```python
from build123d import *

# Parameters (mm, degrees)
PAD_DEPTH       = 10
SKETCH001_R     = 1.75
POCKET_DEPTH    = 15.001
SKETCH002_R     = 4
POCKET001_DEPTH = 5
SKETCH005_R     = 4
SKETCH005_R_2   = 2.25
POCKET002_DEPTH = 9
SKETCH006_W     = 6.5
SKETCH006_H     = 2
POCKET003_DEPTH = 9
FILLET_R        = 3
FILLET001_R     = 3


with BuildPart() as part:
    # Sketch → Pad (new body)
    with BuildSketch(Plane.XY):
        Polygon((-5, 11), (5, 11), (5, -11), (-5, -11), (-10, -2.5), (-10, 2.5), align=None)
    extrude(amount=PAD_DEPTH)

    # Sketch001 → Pocket (cut, through all)
    with BuildSketch(Plane.YZ.offset(5)):
        with Locations((-6, 5)):
            Circle(SKETCH001_R)
        with Locations((6, 5)):
            Circle(SKETCH001_R)
    extrude(amount=-POCKET_DEPTH, mode=Mode.SUBTRACT)

    # Sketch002 → Pocket001 (cut)
    with BuildSketch(Plane(origin=(-10, 0, 0), x_dir=(0, -1, 0), z_dir=(-1, 0, 0))):
        with Locations((-6, 5)):
            Circle(SKETCH002_R)
        with Locations((6, 5)):
            Circle(SKETCH002_R)
    extrude(amount=-POCKET001_DEPTH, mode=Mode.SUBTRACT)

    # Sketch005 → Pocket002 (cut)
    with BuildSketch(Plane.XY.offset(10)):
        Circle(SKETCH005_R)
        Circle(SKETCH005_R_2, mode=Mode.SUBTRACT)
    extrude(amount=-POCKET002_DEPTH, mode=Mode.SUBTRACT)

    # Sketch006 → Pocket003 (cut)
    with BuildSketch(Plane.XY.offset(10)):
        with Locations((-6.75, 0)):
            Rectangle(SKETCH006_W, SKETCH006_H)
    extrude(amount=-POCKET003_DEPTH, mode=Mode.SUBTRACT)

    # Fillet
    fillet_edges = [part.edges().sort_by_distance(p)[0] for p in [
        (-3.872983, 1, 5.5),
    ]]
    fillet(fillet_edges, radius=FILLET_R)

    # Fillet001
    fillet001_edges = [part.edges().sort_by_distance(p)[0] for p in [
        (-3.872983, -1, 5.5),
    ]]
    fillet(fillet001_edges, radius=FILLET001_R)


solid = part.part
```
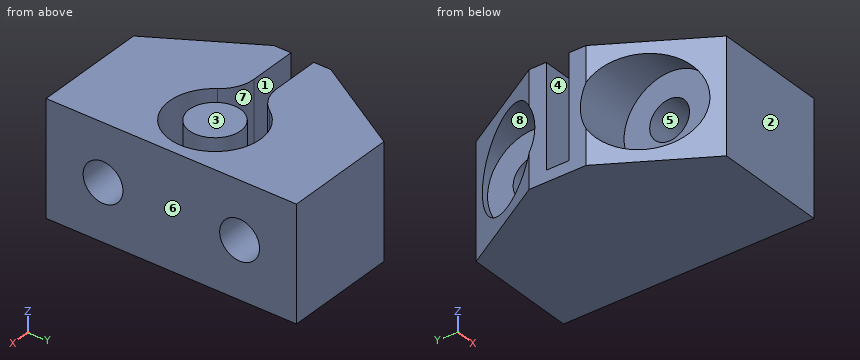
Model file for the job. Use its own axes, mm. Face numbers are marked on the shaded views. A direction names the side the tool comes from. Give positions to 0.01 mm unless a question says otherwise; leave off trailing zeros. Loops run counter-clockwise (first coordinate to the right, second up) from the corner with the lowest first, then second, coordinate; pieces in that order, holes last. Notation, with made-up numbers: (-24.75, 39) - (29.25, 39) arc R29 ccw to (29.25, 69) - close; hole circle Ø11 at (39, 67). An arc over 180 degrees is marked (long way). One line per item, written item: value. Start each with the question number.
1. Pull direction Y, two halves, no side cores. Call the marked faces 1, 2 and 3: pulls with the +Y half, pulls with the -Y half, needs draft (parallel to the pull), parting line crosses it, or undercut.
2. Slice it at C-C (x = -1). List the corners of the cut face in (y, z), plus the area to 3 significant figures.
3. Which spindle directions (+Z, -Z, +X, -X, +Y, -Y) get a long thin tool onto all of the face, cutting with end or side? Do the marked faces 4, 5, 6, 7 and 8. Say none if no direction does.
4. Slice it at D-D (z = 1.25). List the corners of the cut face in (x, y).
5. Slice it at A-A (y = 0). List the corners of the cut face in (x, z).
6. Pin check, flat tips, straight feed: pin 1 (4.5 mm diameter, centred on x = -8.5, z = 7.5, fed in from +Y); pin 2 (3 mm diameter, centred on y = 6, z = 5, fed in from +X); pin 3 (3.5 mm diameter, centred on x = -7, z = 7, fed in from -Y) (3 decimals); pin 4 (5.5 mm diameter, centred on y = -6, z = 5, fed in from -X). Stop position of each tip, or through.
7. Probe L1, parallel to Y at x = -8.2, z = 5; L2, parallel to Y at x = 0.75, z = 6.5; L3, parallel to Z at x = -2.25, y = 6. List the from-to ranges inside material, lowest first. Write a range as from..to.
8. Slice it at B-B (z = 6.5). List the corners of the cut face in (x, y), plus the area to 3 significant figures.
Solution:
1. face 1: undercut
1. face 2: pulls with the -Y half
1. face 3: needs draft
2. outline: (-11, 0) - (11, 0) - (11, 10) - (3.87, 10) - (3.87, 1) - (2.02, 1) - (2.02, 10) - (-2.02, 10) - (-2.02, 1) - (-3.87, 1) - (-3.87, 10) - (-11, 10) - close; hole circle Ø3.5 at (-6, 5); hole circle Ø3.5 at (6, 5)
2. area: 167 mm^2
3. face 4: +Z, -X
3. face 5: +X, -X
3. face 6: +Z, -Z, +X, +Y, -Y
3. face 7: +Z
3. face 8: -X
4. outline: (-10, -2.5) - (-8.76, -4.61) - (-5, -4.61) - (-5, -7.39) - (-7.12, -7.39) - (-5, -11) - (5, -11) - (5, 11) - (-5, 11) - (-7.12, 7.39) - (-5, 7.39) - (-5, 4.61) - (-8.76, 4.61) - (-10, 2.5) - (-10, 1) - (-5.74, 1) arc R3 ccw to (-3.28, 2.29) arc R4 cw (long way) to (-3.28, -2.29) arc R3 ccw to (-5.74, -1) - (-10, -1) - close; circle Ø4.5 at (0, 0)
5. outline: (-10, 0) - (5, 0) - (5, 10) - (4, 10) - (4, 1) - (2.25, 1) - (2.25, 10) - (-2.25, 10) - (-2.25, 1) - (-10, 1) - close
6. pin 1: stops at y = 8.84
6. pin 2: passes through
6. pin 3: stops at y = -10.575
6. pin 4: stops at x = -5
7. L1: y = -2..-1, 1..2
7. L2: y = -11..-6.9, -5.1..-3.93, -2.12..2.12, 3.93..5.1, 6.9..11
7. L3: z = 0..3.25, 6.75..10
8. outline: (-10, -2.29) - (-5, -2.29) - (-5, -5.1) - (5, -5.1) - (5, 5.1) - (-5, 5.1) - (-5, 2.29) - (-10, 2.29) - (-10, 1) - (-5.74, 1) arc R3 ccw to (-3.28, 2.29) arc R4 cw (long way) to (-3.28, -2.29) arc R3 ccw to (-5.74, -1) - (-10, -1) - close; (-5.76, -9.71) - (-5, -11) - (5, -11) - (5, -6.9) - (-5, -6.9) - (-5, -9.71) - close; (-5.76, 9.71) - (-5, 9.71) - (-5, 6.9) - (5, 6.9) - (5, 11) - (-5, 11) - close; circle Ø4.5 at (0, 0)
8. area: 160 mm^2
